The figure shows three views and two pictorial views of one solid part (mm, origin at its lowest corner). Answer the questions. A direction names the side the tool comes from. Coordinates: 2 decimals unless noted, no trailing zeros. Loops run counter-clockwise (first coordinate to the right, second up) from the corner with the lowest first, then second, coordinate; pieces in that order, holes last. Notation, with made-up numbers: M 45,37.5 L 77,37.5 A26 ccw 77,73.5 Z; hole C 85,-0.5 d4. An arc over 180 degrees is marked long. One line per item, written item: value. Start each with the question number.
1. The part is cut by section C-C (x = 43). Write down the section's boundary in (y, z), then the cut area to 3 significant figures.
2. Determine the mould class of the marked faces 3, 4 and 5 for opening direction Y: +Y half, -Y half, draft (parallel to the pull), parting line (faces both ways), or undercut.
3. For the marked faces 1 and 2, determine the directions among +Z, -Z, +X, -X, +Y, -Y from which every point of the face is accessible in a straight line to the end or side of a thin tool.
4. The part is cut by section B-B (z = 35.5). Write down the section's boundary in (x, y).
5. Flat-ended cylindrical pins translate along their axes: pin 1 (19 mm diameter, centred on x = 220, z = 32.5, fed in from +Y); pin 2 (2 mm diameter, centred on x = 188.5, z = 28, fed in from -Y); pin 3 (5 mm diameter, centred on x = 302, y = 4.5, fed in from +Z); pin 4 (5 mm diameter, centred on y = 12, z = 40.5, fed in from +X). Find the tip coordinate at first contact, or state that the pin passes through.
6. The part is cut by section A-A (y = 49). Write down the section's boundary in (x, z), then the cut area to 3 significant figures.
7. The part is cut by section D-D (z = 5). Write down the section's boundary in (x, y), then the cut area to 4 significant figures.
8. Consider probe 1 along Y at (x, z) = (326, 49.5); probe 2 along Y at (x, z) = (166, 17); probe 3 along Y at (x, z) = (139, 47.5). Determine where each line is inside the solid, lowest interval first.
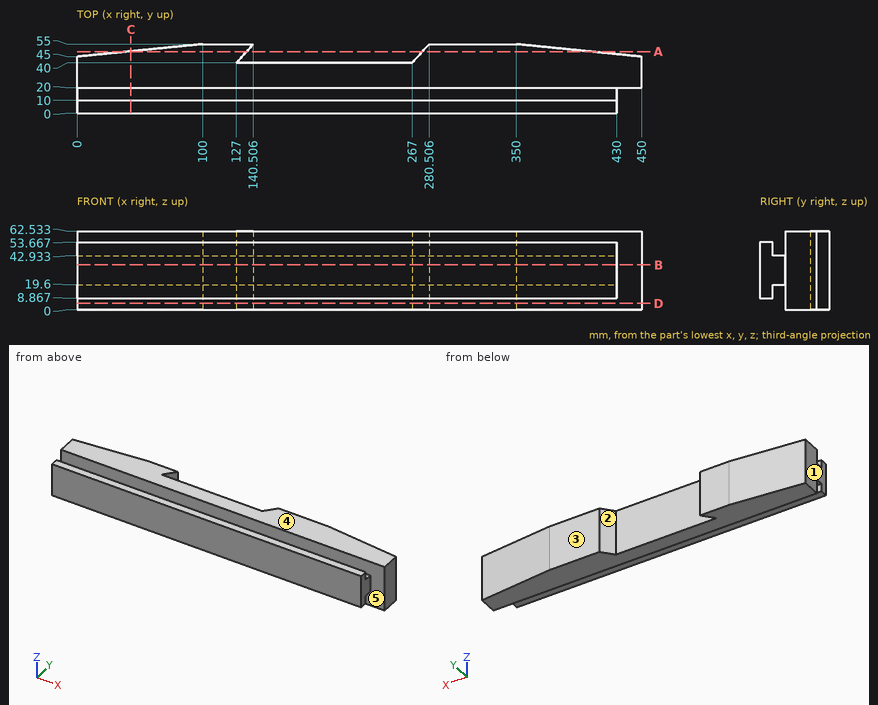
Answer block:
1. outline: M 0,8.87 L 10,8.87 L 10,19.6 L 20,19.6 L 20,0 L 49.3,0 L 49.3,62.53 L 20,62.53 L 20,42.93 L 10,42.93 L 10,53.67 L 0,53.67 Z
1. area: 2,510 mm2
2. face 3: +Y half
2. face 4: draft
2. face 5: undercut
3. face 1: +Z, -Z, -X, +Y, -Y
3. face 2: +Z, -Z, +Y
4. outline: M 0,0 L 430,0 L 430,20 L 450,20 L 450,45 L 350,55 L 280.51,55 L 267,40 L 127,40 L 140.51,55 L 100,55 L 0,45 Z
5. pin 1: stops at y = 40
5. pin 2: stops at y = 0
5. pin 3: stops at z = 53.67
5. pin 4: stops at x = 430
6. outline: M 40,0 L 135.1,0 L 135.1,62.53 L 40,62.53 Z; M 275.1,0 L 410,0 L 410,62.53 L 275.1,62.53 Z
6. area: 14,400 mm2
7. outline: M 0,20 L 450,20 L 450,45 L 350,55 L 280.51,55 L 267,40 L 127,40 L 140.51,55 L 100,55 L 0,45 Z
7. area: 12,650 mm2
8. probe 1: y = 0 to 10, 20 to 55
8. probe 2: y = 0 to 10, 20 to 40
8. probe 3: y = 0 to 10, 20 to 40, 53.33 to 55
